Can you work these out from the model? Positions are in its coordinate system, mm. A direction names the side the tool comes from. Coordinates: 2 decimals unless noted, no trailing zeros. Loops run counter-clockwise (first coordinate to the right, second up) from the corner with the lowest first, then second, coordinate; pieces in that order, holes last.
```python
from build123d import *

# Parameters (mm, degrees)
SKETCH1_W           = 12.5
SKETCH1_H           = 180
BOSS_EXTRUDE1_DEPTH = 20
SKETCH2_R           = 5.65
BOSS_EXTRUDE2_DEPTH = 1.5
SKETCH3_R           = 3.99
BOSS_EXTRUDE3_DEPTH = 7
SKETCH4_R           = 5.65
BOSS_EXTRUDE4_DEPTH = 2.25
SKETCH5_R           = 3.99
BOSS_EXTRUDE5_DEPTH = 7.5
BOSS_EXTRUDE6_START = 2.25
SKETCH6_R           = 5.65
BOSS_EXTRUDE6_DEPTH = 2.25
BOSS_EXTRUDE7_START = 7.5
SKETCH7_R           = 3.99
BOSS_EXTRUDE7_DEPTH = 7.5
SKETCH8_R           = 3.95
CUT_EXTRUDE1_DEPTH  = 19
SKETCH9_W           = 8
SKETCH9_H           = 2
CUT_EXTRUDE2_DEPTH  = 72.5
SKETCH10_W          = 11.5
SKETCH10_H          = 1
CUT_EXTRUDE3_DEPTH  = 72.5
SKETCH11_W          = 12.5
SKETCH11_H          = 21.5
CUT_EXTRUDE4_DEPTH  = 7
CUT_EXTRUDE5_DEPTH  = 20
SKETCH14_W          = 4
SKETCH14_H          = 5
CUT_EXTRUDE6_DEPTH  = 12.5


with BuildPart() as part:
    # Sketch1 → Boss-Extrude1 (new body)
    with BuildSketch(Plane(origin=(0, 0, 0), x_dir=(1, 0, 0), z_dir=(0, 1, 0))):
        Rectangle(SKETCH1_W, SKETCH1_H)
    extrude(amount=BOSS_EXTRUDE1_DEPTH)

    # Sketch2 → Boss-Extrude2 (add)
    with BuildSketch(Plane.XY.offset(90)):
        with Locations(Location((0, 10, 0), (0, 0, 180))):
            Circle(SKETCH2_R)
    extrude(amount=BOSS_EXTRUDE2_DEPTH)

    # Sketch3 → Boss-Extrude3 (add)
    with BuildSketch(Plane.XY.offset(91.5)):
        with Locations(Location((0, 10, 0), (0, 0, 180))):
            Circle(SKETCH3_R)
    extrude(amount=BOSS_EXTRUDE3_DEPTH)

    # Sketch4 → Boss-Extrude4 (add)
    with BuildSketch(Plane.ZY.offset(6.25)):
        with Locations(Location((0, 10, 0), (0, 0, 180))):
            Circle(SKETCH4_R)
    extrude(amount=BOSS_EXTRUDE4_DEPTH)

    # Sketch5 → Boss-Extrude5 (add)
    with BuildSketch(Plane.ZY.offset(8.5)):
        with Locations((0, 10)):
            Circle(SKETCH5_R)
    extrude(amount=BOSS_EXTRUDE5_DEPTH)

    # Sketch6 → Boss-Extrude6 (add)
    with BuildSketch(Plane(origin=(6.25, 0, 0), x_dir=(0, 0, -1), z_dir=(1, 0, 0)).offset(BOSS_EXTRUDE6_START)):
        with Locations((0, 10)):
            Circle(SKETCH6_R)
    extrude(amount=-BOSS_EXTRUDE6_DEPTH)

    # Sketch7 → Boss-Extrude7 (add)
    with BuildSketch(Plane(origin=(8.5, 0, 0), x_dir=(0, 0, -1), z_dir=(1, 0, 0)).offset(BOSS_EXTRUDE7_START)):
        with Locations(Location((0, 10, 0), (0, 0, 180))):
            Circle(SKETCH7_R)
    extrude(amount=-BOSS_EXTRUDE7_DEPTH)

    # Sketch8 → Cut-Extrude1 (cut)
    with BuildSketch(Plane(origin=(0, 20, 0), x_dir=(1, 0, 0), z_dir=(0, 1, 0))):
        with Locations(Location((0, 82.5, 0), (0, 0, 270))):
            Circle(SKETCH8_R)
        with Locations(Location((0, 72.5, 0), (0, 0, 270))):
            Circle(SKETCH8_R)
        with Locations(Location((0, 62.5, 0), (0, 0, 270))):
            Circle(SKETCH8_R)
        with Locations(Location((0, 52.5, 0), (0, 0, 270))):
            Circle(SKETCH8_R)
        with Locations(Location((0, 42.5, 0), (0, 0, 270))):
            Circle(SKETCH8_R)
        with Locations(Location((0, 32.5, 0), (0, 0, 270))):
            Circle(SKETCH8_R)
        with Locations(Location((0, 22.5, 0), (0, 0, 270))):
            Circle(SKETCH8_R)
    extrude(amount=-CUT_EXTRUDE1_DEPTH, mode=Mode.SUBTRACT)

    # Sketch9 → Cut-Extrude2 (cut)
    with BuildSketch(Plane(origin=(0, 0, -90), x_dir=(-1, 0, 0), z_dir=(0, 0, -1))):
        with Locations((0, 18)):
            Rectangle(SKETCH9_W, SKETCH9_H)
    extrude(amount=-CUT_EXTRUDE2_DEPTH, mode=Mode.SUBTRACT)

    # Sketch10 → Cut-Extrude3 (cut)
    with BuildSketch(Plane(origin=(0, 0, -90), x_dir=(-1, 0, 0), z_dir=(0, 0, -1))):
        with Locations((0, 18)):
            Rectangle(SKETCH10_W, SKETCH10_H)
    extrude(amount=-CUT_EXTRUDE3_DEPTH, mode=Mode.SUBTRACT)

    # Sketch11 → Cut-Extrude4 (cut)
    with BuildSketch(Plane(origin=(0, 20, 0), x_dir=(1, 0, 0), z_dir=(0, 1, 0))):
        with Locations((0, -35)):
            Rectangle(SKETCH11_W, SKETCH11_H)
    extrude(amount=-CUT_EXTRUDE4_DEPTH, mode=Mode.SUBTRACT)

    # Sketch12 → Cut-Extrude5 (cut)
    with BuildSketch(Plane.XY.offset(98.5)):
        with BuildLine():
            Line((1.936491673, 10.5), (2.5, 10.5))
            Line((2.5, 10.5), (2.5, 9.5))
            Line((2.5, 9.5), (1.936491673, 9.5))
            ThreePointArc((1.936491673, 9.5), (0, 8), (-1.936491673, 9.5))
            Line((-1.936491673, 9.5), (-2.5, 9.5))
            Line((-2.5, 9.5), (-2.5, 10.5))
            Line((-2.5, 10.5), (-1.936491673, 10.5))
            ThreePointArc((-1.936491673, 10.5), (0, 12), (1.936491673, 10.5))
        make_face()
    extrude(amount=-CUT_EXTRUDE5_DEPTH, mode=Mode.SUBTRACT)

    # Sketch14 → Cut-Extrude6 (cut)
    with BuildSketch(Plane(origin=(6.25, 0, 0), x_dir=(0, 0, -1), z_dir=(1, 0, 0))):
        with Locations((-15, 10)):
            Rectangle(SKETCH14_W, SKETCH14_H)
    extrude(amount=-CUT_EXTRUDE6_DEPTH, mode=Mode.SUBTRACT)


solid = part.part
```
(1) Which directions (+Z, -Z, +X, -X, +Y, -Y) give clear straight access to the entire face, cutting with the end or side of a thin tool? Please do faces 5 (the flat face through (3.6, 19, -70.4)), 6 (the flat face through (0, 0, -1)), 7 (the flat face through (0, 1, -53)), 8 (the flat face through (0, 10, 13)), 9 (the flat face through (0, 10, -90)).
Check values:
face 5: -Z
face 6: +Z, -Z, +X, -X, -Y
face 7: +Y
face 8: +X, -X
face 9: -Z, +X, -X, +Y, -Y
(2) If I drill on probe 1 along Y at (x, z) = (4.5, -49); probe 2 along X at (y, z) = (19.45, -62.5); probe 3 along X at (y, z) = (11.75, 9.5), over which ranges is the centre line in solid material (lowest first)?
Check values:
probe 1: y = 0 to 17.5, 18.5 to 20
probe 2: x = -6.25 to -3.95, 3.95 to 6.25
probe 3: x = -6.25 to 6.25
(3) If we mould it in two halves opening along X, with no side actions, what happens to faces 1 (the flat face through (0, 7.5, 15)), 2 (the cylindrical face through (0, 12, 89)), 3 (the flat face through (8.5, 6, -2)), 4 (the cylindrical face through (0.174, 9.112, -66.446))? For each: released by +X, released by -X, zero draft, split by the parting line, or undercut.
Check values:
face 1: zero draft
face 2: undercut
face 3: released by +X
face 4: undercut
(4) I want a section at B-B on x = 0. State how many separate pieces and enclosed holes the cut face has, then the cut area to 3 significant figures.
Check values:
separate pieces: 8
enclosed holes: 1
area: 2,340 mm2
(5) I want a section at C-C on x = 13. Write out the boundary of the cut face in (y, z).
Check values:
outline: circle Ø7.98 at (10, 0)
(6) I want a section at D-D on z = 0. Write out the boundary of the cut face in (x, y), then the cut area to 3 significant figures.
Check values:
outline: (-16, 6.01) - (-8.5, 6.01) - (-8.5, 4.35) - (-6.25, 4.35) - (-6.25, 0) - (6.25, 0) - (6.25, 4.35) - (8.5, 4.35) - (8.5, 6.01) - (16, 6.01) - (16, 13.99) - (8.5, 13.99) - (8.5, 15.65) - (6.25, 15.65) - (6.25, 20) - (-6.25, 20) - (-6.25, 15.65) - (-8.5, 15.65) - (-8.5, 13.99) - (-16, 13.99) - close
area: 421 mm2
(7) I want a section at A-A on z = -22.5. Write out the boundary of the cut face in (x, y), then the cut area to 3 significant figures.
Check values:
outline: (-6.25, 0) - (6.25, 0) - (6.25, 20) - (3.95, 20) - (3.95, 19) - (4, 19) - (4, 18.5) - (5.75, 18.5) - (5.75, 17.5) - (4, 17.5) - (4, 17) - (3.95, 17) - (3.95, 1) - (-3.95, 1) - (-3.95, 17) - (-4, 17) - (-4, 17.5) - (-5.75, 17.5) - (-5.75, 18.5) - (-4, 18.5) - (-4, 19) - (-3.95, 19) - (-3.95, 20) - (-6.25, 20) - close
area: 96.2 mm2
(8) I'm going to push flat-ended pins straight in: pin 1 (4 mm diameter, centred on x = 4, z = -25.5, fed in from -Y); pin 2 (2 mm diameter, centred on x = 8.5, y = 9.5, fed in from -Z); pin 3 (2.5 mm diameter, centred on x = 1, z = -33.5, fed in from +Y); pin 4 (10 mm diameter, centred on y = 12, z = -51.5, fed in from +X). Where does each tip first touch, or does it pass through?
Check values:
pin 1: stops at y = 0
pin 2: stops at z = -5.65
pin 3: stops at y = 1
pin 4: stops at x = 6.25
